Study the drawing (mm; zero at the part's minimum x, y, z) and answer. A direction names the side the tool comes from. Give positions to 0.01 mm unless a question says otherwise; leave off trailing zeros. Loops run counter-clockwise (first coordinate to the right, second up) from the corner with the lowest first, then second, coordinate; pieces in that order, holes last. Notation, with made-up numbers: M -14.5,64.5 L 35.5,64.5 A12 ccw 35.5,77.5 Z; hole C 71,-16.5 d6. An arc over 180 degrees is marked long. Use one line per item in the form item = value. Start each with the question number.
1. The part is cut by section B-B (y = 10). Write down the section's boundary in (x, z) (1 decimal), and give its area (3 significant figures).
2. The part is cut by section C-C (z = 12). Write down the section's boundary in (x, y), and give its area (3 significant figures).
3. Straight lines are drawn through the part: line 1 (Z direction, x = 18, y = 7.75); line 2 (Y direction, x = 36, z = 15); line 3 (Z direction, x = 7, y = 9.75) (1 decimal). For each, find the intervals that lie inside material, in ascending order. Write a range as from..to.
4. For the marked faces 1, 2 and 3, determine the directions among +Z, -Z, +X, -X, +Y, -Y from which every point of the face is accessible in a straight line to the end or side of a thin tool.
5. The mould has two halves that part along X. Classify the marked faces 4, 5 and 6: released by +X, released by -X, zero draft, split by the parting line, or undercut.
6. Each of these flat-tipped pins is pushed along its axis until it touches: pin 1 Ø5 at (x, z) = (31.5, 8) entering from -Y; pin 2 Ø4 at (x, y) = (20.5, 4.5) entering from +Z; pin 3 Ø7.5 at (x, z) = (29.5, 9.5) entering from +Y. Where does it stop, or does it pass through?
7. The part is cut by section D-D (z = 9). Write down the section's boundary in (x, y) (1 decimal).
8. The part is cut by section A-A (x = 38.5). Write down the section's boundary in (y, z) (1 decimal).
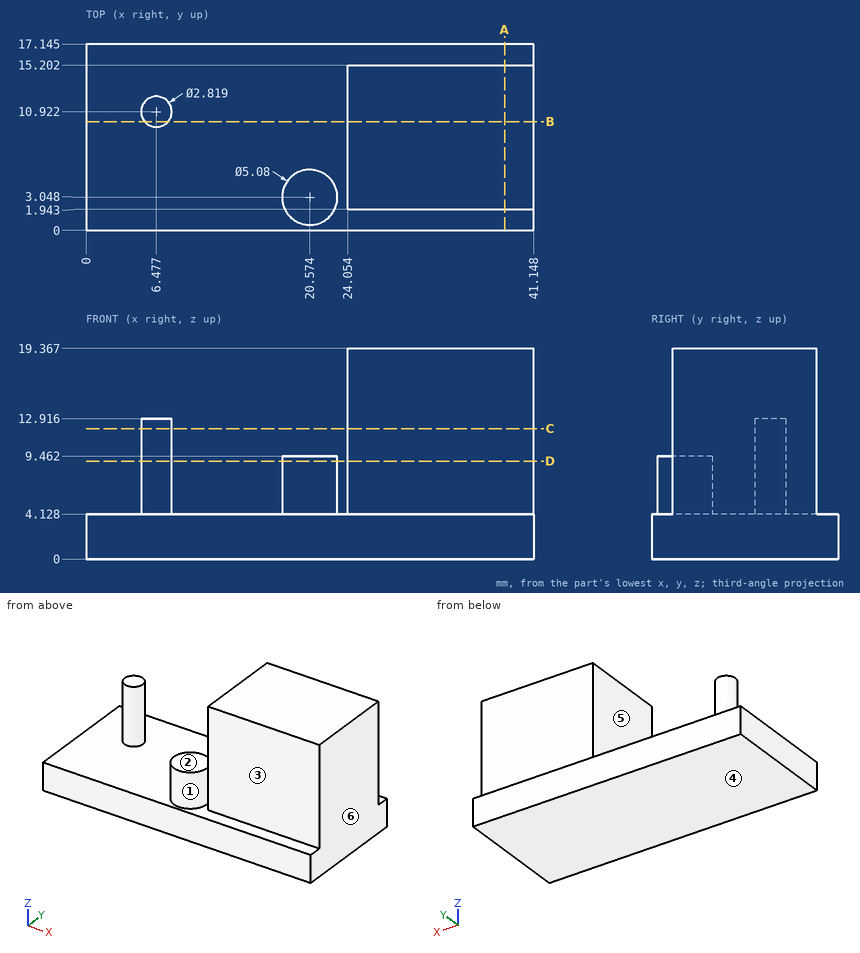
Derived:
q1.outline = M 0,0 L 41.1,0 L 41.1,19.4 L 24.1,19.4 L 24.1,4.1 L 7.5,4.1 L 7.5,12.9 L 5.4,12.9 L 5.4,4.1 L 0,4.1 Z
q1.area = 449 mm2
q2.outline = C 6.48,10.92 d2.82; M 24.05,1.94 L 41.15,1.94 L 41.15,15.2 L 24.05,15.2 Z
q2.area = 233 mm2
q3.line_1 = 0..4.13
q3.line_2 = 1.94..15.2
q3.line_3 = 0..12.9
q4.face_1 = +Z
q4.face_2 = +Z, -X, +Y, -Y
q4.face_3 = +Z, +X, -Y
q5.face_4 = zero draft
q5.face_5 = undercut
q5.face_6 = released by +X
q6.pin_1 = 1.94
q6.pin_2 = 9.46
q6.pin_3 = 15.2
q7.outline = C 6.5,10.9 d2.8; C 20.6,3 d5.1; M 24.1,1.9 L 41.1,1.9 L 41.1,15.2 L 24.1,15.2 Z
q8.outline = M 0,0 L 17.1,0 L 17.1,4.1 L 15.2,4.1 L 15.2,19.4 L 1.9,19.4 L 1.9,4.1 L 0,4.1 Z
